from build123d import *

# Parameters (mm, degrees)
SKETCH1_W           = 80
SKETCH1_H           = 108
SKETCH1_R           = 16
SKETCH1_R_2         = 11
SKETCH1_R_3         = 2.1
SKETCH1_R_4         = 1.25
SKETCH1_R_5         = 2.5
BOSS_EXTRUDE1_DEPTH = 2.5
FILLET1_R           = 5


with BuildPart() as part:
    # Sketch1 → Boss-Extrude1 (new, symmetric)
    with BuildSketch(Plane.XY):
        Rectangle(SKETCH1_W, SKETCH1_H)
        with Locations((0, -24)):
            Circle(SKETCH1_R, mode=Mode.SUBTRACT)
        with Locations((0, 34.6)):
            Circle(SKETCH1_R_2, mode=Mode.SUBTRACT)
        with Locations((21, -24)):
            Circle(SKETCH1_R_3, mode=Mode.SUBTRACT)
        with Locations((-21, -24)):
            Circle(SKETCH1_R_3, mode=Mode.SUBTRACT)
        with Locations((0, -3)):
            Circle(SKETCH1_R_3, mode=Mode.SUBTRACT)
        with Locations((0, -45)):
            Circle(SKETCH1_R_3, mode=Mode.SUBTRACT)
        with Locations((15.5, 50.1)):
            Circle(SKETCH1_R_4, mode=Mode.SUBTRACT)
        with Locations((15.5, 19.1)):
            Circle(SKETCH1_R_4, mode=Mode.SUBTRACT)
        with Locations((-15.5, 19.1)):
            Circle(SKETCH1_R_4, mode=Mode.SUBTRACT)
        with Locations((-15.5, 50.1)):
            Circle(SKETCH1_R_4, mode=Mode.SUBTRACT)
        with Locations((25.5, -45.5)):
            Circle(SKETCH1_R_5, mode=Mode.SUBTRACT)
        with Locations((-25.5, -45.5)):
            Circle(SKETCH1_R_5, mode=Mode.SUBTRACT)
        with Locations((-25.5, -2.5)):
            Circle(SKETCH1_R_5, mode=Mode.SUBTRACT)
        with Locations((25.5, -2.5)):
            Circle(SKETCH1_R_5, mode=Mode.SUBTRACT)
        with BuildLine():
            Line((31.5, -46.5), (31.5, -44.5))
            ThreePointArc((31.5, -44.5), (33, -43), (34.5, -44.5))
            Line((34.5, -44.5), (34.5, -46.5))
            ThreePointArc((34.5, -46.5), (33, -48), (31.5, -46.5))
        make_face(mode=Mode.SUBTRACT)
        with BuildLine():
            Line((-31.5, -46.5), (-31.5, -44.5))
            ThreePointArc((-31.5, -44.5), (-33, -43), (-34.5, -44.5))
            Line((-34.5, -44.5), (-34.5, -46.5))
            ThreePointArc((-34.5, -46.5), (-33, -48), (-31.5, -46.5))
        make_face(mode=Mode.SUBTRACT)
        with BuildLine():
            Line((-15.5, -46.5), (-15.5, -44.5))
            ThreePointArc((-15.5, -44.5), (-17, -43), (-18.5, -44.5))
            Line((-18.5, -44.5), (-18.5, -46.5))
            ThreePointArc((-18.5, -46.5), (-17, -48), (-15.5, -46.5))
        make_face(mode=Mode.SUBTRACT)
        with BuildLine():
            Line((15.5, -46.5), (15.5, -44.5))
            ThreePointArc((15.5, -44.5), (17, -43), (18.5, -44.5))
            Line((18.5, -44.5), (18.5, -46.5))
            ThreePointArc((18.5, -46.5), (17, -48), (15.5, -46.5))
        make_face(mode=Mode.SUBTRACT)
        with BuildLine():
            Line((-31.5, -1.5), (-31.5, -3.5))
            ThreePointArc((-31.5, -3.5), (-33, -5), (-34.5, -3.5))
            Line((-34.5, -3.5), (-34.5, -1.5))
            ThreePointArc((-34.5, -1.5), (-33, 0), (-31.5, -1.5))
        make_face(mode=Mode.SUBTRACT)
        with BuildLine():
            Line((-15.5, -1.5), (-15.5, -3.5))
            ThreePointArc((-15.5, -3.5), (-17, -5), (-18.5, -3.5))
            Line((-18.5, -3.5), (-18.5, -1.5))
            ThreePointArc((-18.5, -1.5), (-17, 0), (-15.5, -1.5))
        make_face(mode=Mode.SUBTRACT)
        with BuildLine():
            Line((31.5, -1.5), (31.5, -3.5))
            ThreePointArc((31.5, -3.5), (33, -5), (34.5, -3.5))
            Line((34.5, -3.5), (34.5, -1.5))
            ThreePointArc((34.5, -1.5), (33, 0), (31.5, -1.5))
        make_face(mode=Mode.SUBTRACT)
        with BuildLine():
            Line((15.5, -1.5), (15.5, -3.5))
            ThreePointArc((15.5, -3.5), (17, -5), (18.5, -3.5))
            Line((18.5, -3.5), (18.5, -1.5))
            ThreePointArc((18.5, -1.5), (17, 0), (15.5, -1.5))
        make_face(mode=Mode.SUBTRACT)
        with BuildLine():
            Line((8.170175088, 8.634889115), (24.144949642, 14.449231552))
            ThreePointArc((24.144949642, 14.449231552), (27.349231552, 12.955050358), (25.855050358, 9.750768448))
            Line((25.855050358, 9.750768448), (9.880275805, 3.936426011))
            ThreePointArc((9.880275805, 3.936426011), (6.675993895, 5.430607205), (8.170175088, 8.634889115))
        make_face(mode=Mode.SUBTRACT)
    extrude(amount=BOSS_EXTRUDE1_DEPTH, both=True)

    # Fillet1
    fillet1_edges = [part.edges().sort_by_distance(p)[0] for p in [
        (40, -54, 0),
        (-40, -54, 0),
        (-40, 54, 0),
        (40, 54, 0),
    ]]
    fillet(fillet1_edges, radius=FILLET1_R)


solid = part.part
Verification items for the finished model (mm, model axes). A direction names the side the tool comes from. Round coordinates to 2 decimals unless told otherwise and drop trailing zeros. Loops run counter-clockwise (first coordinate to the right, second up) from the corner with the lowest first, then second, coordinate; pieces in that order, holes last. Notation, with made-up numbers: (28, -3.5) - (73, -3.5) arc R33 cw to (73, 26.5) - close; hole circle Ø4 at (22, 55.25). An arc over 180 degrees is marked (long way). Write item = value, one per line.
Q1. Sectioned sample at A-A on x = 0. Record the boundary of the cut face in (y, z).
Here are the results:
outline = (-54, -2.5) - (-47.1, -2.5) - (-47.1, 2.5) - (-54, 2.5) - close; (-42.9, -2.5) - (-40, -2.5) - (-40, 2.5) - (-42.9, 2.5) - close; (-8, -2.5) - (-5.1, -2.5) - (-5.1, 2.5) - (-8, 2.5) - close; (-0.9, -2.5) - (23.6, -2.5) - (23.6, 2.5) - (-0.9, 2.5) - close; (45.6, -2.5) - (54, -2.5) - (54, 2.5) - (45.6, 2.5) - close
Q2. Sectioned sample at D-D on y = 43.5. Record the boundary of the cut face in (x, z), plus the area to 3 significant figures.
Here are the results:
outline = (-40, -2.5) - (-6.46, -2.5) - (-6.46, 2.5) - (-40, 2.5) - close; (6.46, -2.5) - (40, -2.5) - (40, 2.5) - (6.46, 2.5) - close
area = 335 mm^2
Q3. Mould release check, pull along X, two halves, no side actions. Record for faces 1 (the flat face through (0, 54, 0)), 2 (the cylindrical face through (-17, 0, 0)), 3 (the flat face through (40, -1, 0)): +X half, -X half, draft (parallel to the pull), parting line (faces both ways), or undercut.
Here are the results:
face_1 = draft
face_2 = undercut
face_3 = +X half
Q4. Sectioned sample at B-B on y = -24. Record the boundary of the cut face in (x, z), plus the area to 3 significant figures.
Here are the results:
outline = (-40, -2.5) - (-23.1, -2.5) - (-23.1, 2.5) - (-40, 2.5) - close; (-18.9, -2.5) - (-16, -2.5) - (-16, 2.5) - (-18.9, 2.5) - close; (16, -2.5) - (18.9, -2.5) - (18.9, 2.5) - (16, 2.5) - close; (23.1, -2.5) - (40, -2.5) - (40, 2.5) - (23.1, 2.5) - close
area = 198 mm^2
Q5. Material ranges on L1, parallel to Y at x = 0, z = 0.1; L2, parallel to Y at x = -25.5, z = 1.15; L3, parallel to Y at x = 4.5, z = -0.25, recorded low to high.
Here are the results:
L1 = -54 to -47.1, -42.9 to -40, -8 to -5.1, -0.9 to 23.6, 45.6 to 54
L2 = -54 to -48, -43 to -5, 0 to 54
L3 = -54 to -39.35, -8.65 to 24.56, 44.64 to 54
Q6. Tool access check on faces 4 (the cylindrical face through (-39, 52, 0)), 5 (the cylindrical face through (-33, -5, 0)). Record the directions out of +Z, -Z, +X, -X, +Y, -Y that give a thin tool (end or side, any length) a straight path to the whole face; none if there is none.
Here are the results:
face_4 = +Z, -Z, -X, +Y
face_5 = +Z, -Z
Q7. Sectioned sample at C-C on x = 33. Record the boundary of the cut face in (y, z), plus the area to 3 significant figures.
Here are the results:
outline = (-54, -2.5) - (-48, -2.5) - (-48, 2.5) - (-54, 2.5) - close; (-43, -2.5) - (-5, -2.5) - (-5, 2.5) - (-43, 2.5) - close; (0, -2.5) - (54, -2.5) - (54, 2.5) - (0, 2.5) - close
area = 490 mm^2
